CAD build for the part. Positions are in the model's coordinates, mm. A direction names the side the tool comes from. Coordinates: 2 decimals unless noted, no trailing zeros. Loops run counter-clockwise (first coordinate to the right, second up) from the corner with the lowest first, then second, coordinate; pieces in that order, holes last.
1) Two-plate mould, pull along X, no slides. Class faces 1 (the cylindrical face through (-6.64, -2.4, -98.38)), 2 (the flat face through (5.5, 2, -51)), 3 (the flat face through (10, -23, -16)), 4 (the flat face through (-10, -23, -16)): +X half, -X half, draft (parallel to the pull), parting line (faces both ways), or undercut.
2) Wall check: line 1 along X through (y, z) = (0, -3); line 2 along X through (y, z) = (40.5, -69); line 3 along Z through (x, y) = (-3.25, -9.5). Give the ranges that are in metal, low to high.
3) Pin check, flat tips, straight feed: pin 1 Ø20.5 at (y, z) = (-2.5, -37.5) entering from +X; pin 2 Ø3.5 at (x, z) = (0, -48.5) entering from +Y (3 decimals); pin 3 Ø2.5 at (x, y) = (0, 0) entering from -Z; pin 4 Ø4 at (x, z) = (0, -94.04) entering from +Y. Stop position of each tip, or through.
4) Saw through at A-A, the plane z = -50.8. Write the cut outline in (x, y) (3 decimals), and give its area (3 significant figures).
5) Which spindle directions (+Z, -Z, +X, -X, +Y, -Y) get a long thin tool onto all of the face, cutting with end or side? Do faces 5 (the cylindrical face through (6.8, 46.94, -3.65)), 6 (the cylindrical face through (-3.858, 0.108, -3.219)), 7 (the conical face through (4.67, -0.16, -94.03)). Say none if no direction does.
```python
from build123d import *

# Parameters (mm, degrees)
SKETCH1_W                        = 20
SKETCH1_H                        = 101.6
BOSS_EXTRUDE1_DEPTH              = 101.6
SKETCH3_W                        = 11
SKETCH3_H                        = 68.58
CUT_EXTRUDE1_DEPTH               = 98.425
CUT_EXTRUDE2_REACH               = 116.032
SKETCH4_W                        = 3
SKETCH4_H                        = 98.425
SKETCH5_R                        = 40.64
CUT_EXTRUDE3_DEPTH               = 2.5
CUT_EXTRUDE3_DRAFT               = -45
SKETCH6_R                        = 40.64
CUT_EXTRUDE4_DEPTH               = 2.5
CUT_EXTRUDE4_DRAFT               = -45
F_10_0_1935_DIAMETER_HOLE1_D     = 4.9149
F_10_0_1935_DIAMETER_HOLE1_DEPTH = 7.62
F_10_0_1935_DIAMETER_HOLE1_TIP   = 1.476584928
CUT_EXTRUDE5_REACH               = 116.032
SKETCH9_R                        = 1.5
F_10_0_1935_DIAMETER_HOLE2_D     = 4.9149
F_10_0_1935_DIAMETER_HOLE2_DEPTH = 6.35
F_10_0_1935_DIAMETER_HOLE2_TIP   = 1.476584928
F_10_0_1935_DIAMETER_HOLE3_D     = 4.9149
F_10_0_1935_DIAMETER_HOLE3_DEPTH = 6.35
F_10_0_1935_DIAMETER_HOLE3_TIP   = 1.476584928


with BuildPart() as part:
    # Sketch1 → Boss-Extrude1 (new body)
    with BuildSketch(Plane.XY):
        Rectangle(SKETCH1_W, SKETCH1_H)
    extrude(amount=-BOSS_EXTRUDE1_DEPTH)

    # Sketch3 → Cut-Extrude1 (cut)
    with BuildSketch(Plane(origin=(0, 50.8, 0), x_dir=(1, 0, 0), z_dir=(0, 1, 0))):
        with Locations((0, 51.7525)):
            Rectangle(SKETCH3_W, SKETCH3_H)
    extrude(amount=-CUT_EXTRUDE1_DEPTH, mode=Mode.SUBTRACT)

    # Sketch4 → Cut-Extrude2 (cut, up to next)
    with BuildSketch(Plane.XY, mode=Mode.PRIVATE) as cut_extrude2_sk1:
        with Locations((0, 1.5875)):
            Rectangle(SKETCH4_W, SKETCH4_H)
    cut_extrude2_tool1 = extrude(cut_extrude2_sk1.sketch, amount=-CUT_EXTRUDE2_REACH, mode=Mode.PRIVATE) & part.part
    add(cut_extrude2_tool1.solids().sort_by_distance((0, 1.5875, 0))[0], mode=Mode.SUBTRACT)


with BuildPart() as cut_extrude3_tool:
    # Sketch5 → Cut-Extrude3 (with draft: the straight prism first)
    with BuildSketch(Plane(origin=(10, 0, 0), x_dir=(0, 0, -1), z_dir=(1, 0, 0))):
        with Locations((50.8, 0)):
            Circle(SKETCH5_R)
    extrude(amount=-CUT_EXTRUDE3_DEPTH)
    # Cut-Extrude3: the draft: its side faces are tilted about the plane it starts from
    cut_extrude3_sides = [cut_extrude3_tool.faces().sort_by_distance(p)[0] for p in [
        (8.75, 0, -10.16),
    ]]
    draft(cut_extrude3_sides, Plane(origin=(10, 0, 0), x_dir=(0, 0, -1), z_dir=(1, 0, 0)), CUT_EXTRUDE3_DRAFT)


with BuildPart() as part_1:
    add(part.part)

    # Cut-Extrude3: cut by cut_extrude3_tool
    add(cut_extrude3_tool.part, mode=Mode.SUBTRACT)


with BuildPart() as cut_extrude4_tool:
    # Sketch6 → Cut-Extrude4 (with draft: the straight prism first)
    with BuildSketch(Plane.ZY.offset(10)):
        with Locations((-50.8, 0)):
            Circle(SKETCH6_R)
    extrude(amount=-CUT_EXTRUDE4_DEPTH)
    # Cut-Extrude4: the draft: its side faces are tilted about the plane it starts from
    cut_extrude4_sides = [cut_extrude4_tool.faces().sort_by_distance(p)[0] for p in [
        (-8.75, 0, -91.44),
    ]]
    draft(cut_extrude4_sides, Plane.ZY.offset(10), CUT_EXTRUDE4_DRAFT)


with BuildPart() as part_2:
    add(part_1.part)

    # Cut-Extrude4: cut by cut_extrude4_tool
    add(cut_extrude4_tool.part, mode=Mode.SUBTRACT)

    # #10 (0.1935) Diameter Hole1
    with Locations(Plane(origin=(0, 50.8, 0), x_dir=(1, 0, 0), z_dir=(0, 1, 0))):
        with Locations((-5.494388528, 6.046802712), (6.262656147, 6.046802712), (0, 94.038956273)):
            Hole(F_10_0_1935_DIAMETER_HOLE1_D / 2, depth=F_10_0_1935_DIAMETER_HOLE1_DEPTH)
            with Locations((0, 0, -(F_10_0_1935_DIAMETER_HOLE1_DEPTH + F_10_0_1935_DIAMETER_HOLE1_TIP / 2))):  # 118° drill point
                Cone(0, F_10_0_1935_DIAMETER_HOLE1_D / 2, F_10_0_1935_DIAMETER_HOLE1_TIP, mode=Mode.SUBTRACT)

    # Sketch9 → Cut-Extrude5 (cut, up to next)
    with BuildSketch(Plane(origin=(0, 0, -101.6), x_dir=(-1, 0, 0), z_dir=(0, 0, -1)), mode=Mode.PRIVATE) as cut_extrude5_sk1:
        Circle(SKETCH9_R)
    cut_extrude5_tool1 = extrude(cut_extrude5_sk1.sketch, amount=-CUT_EXTRUDE5_REACH, mode=Mode.PRIVATE) & part_2.part
    add(cut_extrude5_tool1.solids().sort_by_distance((0, 0, -101.6))[0], mode=Mode.SUBTRACT)

    # #10 (0.1935) Diameter Hole2
    with Locations(Plane.XY):
        with Locations((4.80953422, 0), (-6.312598241, 0)):
            Hole(F_10_0_1935_DIAMETER_HOLE2_D / 2, depth=F_10_0_1935_DIAMETER_HOLE2_DEPTH)
            with Locations((0, 0, -(F_10_0_1935_DIAMETER_HOLE2_DEPTH + F_10_0_1935_DIAMETER_HOLE2_TIP / 2))):  # 118° drill point
                Cone(0, F_10_0_1935_DIAMETER_HOLE2_D / 2, F_10_0_1935_DIAMETER_HOLE2_TIP, mode=Mode.SUBTRACT)

    # #10 (0.1935) Diameter Hole3
    with Locations(Plane(origin=(0, 0, -101.6), x_dir=(-1, 0, 0), z_dir=(0, 0, -1))):
        with Locations((6.103302253, 0), (-5.068844244, 0)):
            Hole(F_10_0_1935_DIAMETER_HOLE3_D / 2, depth=F_10_0_1935_DIAMETER_HOLE3_DEPTH)
            with Locations((0, 0, -(F_10_0_1935_DIAMETER_HOLE3_DEPTH + F_10_0_1935_DIAMETER_HOLE3_TIP / 2))):  # 118° drill point
                Cone(0, F_10_0_1935_DIAMETER_HOLE3_D / 2, F_10_0_1935_DIAMETER_HOLE3_TIP, mode=Mode.SUBTRACT)


solid = part_2.part
```
Data:
1. face 1: undercut
1. face 2: undercut
1. face 3: +X half
1. face 4: -X half
2. line 1: x = -10 to -8.77, -3.86 to -1.5, 1.5 to 2.35, 7.27 to 10
2. line 2: x = -10 to -5.5, 5.5 to 10
2. line 3: z = -101.6 to -86.04, -17.46 to 0
3. pin 1: stops at x = 7.5
3. pin 2: stops at y = -47.625
3. pin 3: passes through
3. pin 4: stops at y = 42.91
4. outline: (-10, -50.8) - (10, -50.8) - (10, -40.64) - (7.5, -38.14) - (7.5, 38.14) - (10, 40.64) - (10, 50.8) - (5.5, 50.8) - (5.5, -47.625) - (-5.5, -47.625) - (-5.5, 50.8) - (-10, 50.8) - (-10, 40.64) - (-7.5, 38.14) - (-7.5, -38.14) - (-10, -40.64) - close
4. area: 555 mm2
5. face 5: +Y
5. face 6: +Z
5. face 7: -Z
